```python
from build123d import *

# Parameters (mm, degrees)
F0_W     = 48.9
F0_H     = 26.2
F1_DEPTH = 1
F2_SIZE  = 4
F3_W     = 6
F3_H     = 8
F4_DEPTH = 3


with BuildPart() as f1:
    # F0 (on Top) → F1 (new body)
    with BuildSketch(Plane.XY):
        Rectangle(F0_W, F0_H)
    extrude(amount=F1_DEPTH)

    # F2
    f2_edges = [f1.edges().sort_by_distance(p)[0] for p in [
        (24.45, 13.1, 0.5),
        (24.45, -13.1, 0.5),
    ]]
    chamfer(f2_edges, length=F2_SIZE)

    # F3 (on face) → F4 (join)
    with BuildSketch(Plane.XY.offset(1)):
        with Locations((-21.45, 0)):
            Rectangle(F3_W, F3_H)
    extrude(amount=F4_DEPTH)


solid = f1.part
```
For this review, take the finished solid that the model builds, in its own axes (mm). A direction names the side the tool comes from. Round coordinates to 2 decimals unless told otherwise and drop trailing zeros. Write each loop counter-clockwise with the first axis right and the second up, starting at its lowest first coordinate (ties: lowest second). Pieces come first, ordered by that corner, then holes. Notation, with made-up numbers: (0, -25) -> (28, -25) arc R6 cw to (28, -15) -> close; hole circle Ø10 at (-30.5, 46.5). An arc over 180 degrees is marked (long way). One line per question, with ' | ' between items. Start each with the question number.
1) Machinability: for faces 1 (the flat face through (-21, 4, 2)), 2 (the flat face through (-2.3, 13.1, 0.5)), 3 (the flat face through (-18.45, 0, 2)), 4 (the flat face through (-21, -4, 2)), which of the approach directions +Z, -Z, +X, -X, +Y, -Y give a long, thin tool a straight path to every point of the face, cutting with its end or side? Answer none if there is none.
2) Wall thickness on line 1 along Z through (x, y) = (-3.5, -8.5); line 2 along X through (y, z) = (-3, 2.3): over which ranges is each line inside the solid? List them lowest first.
3) Add section B-B (y = 10). Write out the cut boundary in (x, z), and give its area (3 significant figures).
4) For pin 1 Ø1.5 at (x, y) = (2, 8.5) entering from +Z; pin 2 Ø1.5 at (y, z) = (1, 2.5) entering from +X; pin 3 Ø0.9 at (x, z) = (-22, 2) entering from +Y, all flat-tipped, find the tip position at first contact; note any pin that passes through.
5) Add section C-C (y = -3). Write out the cut boundary in (x, z).
6) Add section A-A (z = 2.5). Write out the cut boundary in (x, y).
Reported:
1) face 1: +Z, +X, -X, +Y | face 2: +Z, -Z, +X, -X, +Y | face 3: +Z, +X, +Y, -Y | face 4: +Z, +X, -X, -Y
2) line 1: z = 0 to 1 | line 2: x = -24.45 to -18.45
3) outline: (-24.45, 0) -> (23.55, 0) -> (23.55, 1) -> (-24.45, 1) -> close | area: 48.0 mm²
4) pin 1: stops at z = 1 | pin 2: stops at x = -18.45 | pin 3: stops at y = 4
5) outline: (-24.45, 0) -> (24.45, 0) -> (24.45, 1) -> (-18.45, 1) -> (-18.45, 4) -> (-24.45, 4) -> close
6) outline: (-24.45, -4) -> (-18.45, -4) -> (-18.45, 4) -> (-24.45, 4) -> close
